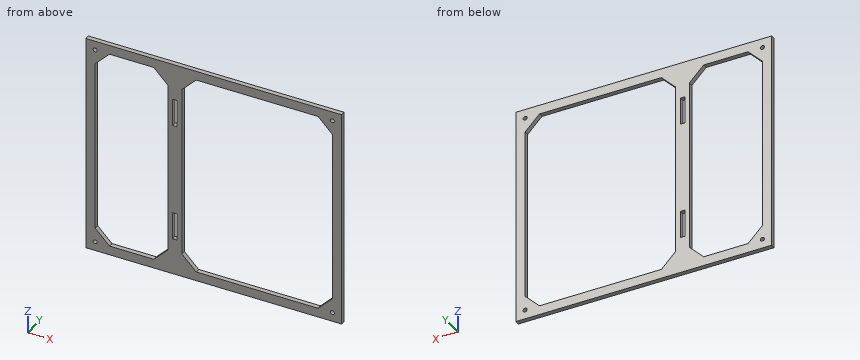
from build123d import *

# Parameters (mm, degrees)
SKETCH1_W           = 177.8
SKETCH1_H           = 152.4
SKETCH1_R           = 1.375
SKETCH1_W_2         = 3.175
SKETCH1_H_2         = 19.05
BOSS_EXTRUDE5_DEPTH = 3.175


with BuildPart() as part:
    # Sketch1 → Boss-Extrude5 (new body)
    with BuildSketch(Plane(origin=(0, 0, 0), x_dir=(1, 0, 0), z_dir=(0, 1, 0))):
        with Locations((88.9, 76.2)):
            Rectangle(SKETCH1_W, SKETCH1_H)
        with Locations(Location((6.35, 146.05, 0), (0, 0, 270))):
            Circle(SKETCH1_R, mode=Mode.SUBTRACT)
        with Locations(Location((6.35, 6.35, 0), (0, 0, 270))):
            Circle(SKETCH1_R, mode=Mode.SUBTRACT)
        with Locations(Location((171.45, 6.35, 0), (0, 0, 270))):
            Circle(SKETCH1_R, mode=Mode.SUBTRACT)
        with Locations(Location((171.45, 146.05, 0), (0, 0, 270))):
            Circle(SKETCH1_R, mode=Mode.SUBTRACT)
        Polygon((6.35, 16.35), (16.35, 6.35), (47.15, 6.35), (57.15, 16.35), (57.15, 136.05), (47.15, 146.05), (16.35, 146.05), (6.35, 136.05), align=None, mode=Mode.SUBTRACT)
        Polygon((76.675, 146.05), (161.45, 146.05), (171.45, 136.05), (171.45, 16.35), (161.45, 6.35), (76.675, 6.35), (66.675, 16.35), (66.675, 136.05), align=None, mode=Mode.SUBTRACT)
        with Locations((61.9125, 117.475)):
            Rectangle(SKETCH1_W_2, SKETCH1_H_2, mode=Mode.SUBTRACT)
        with Locations((61.9125, 34.925)):
            Rectangle(SKETCH1_W_2, SKETCH1_H_2, mode=Mode.SUBTRACT)
    extrude(amount=BOSS_EXTRUDE5_DEPTH)


solid = part.part
Model file for the job. Use its own axes, mm. Give positions to 0.01 mm unless a question says otherwise; leave off trailing zeros. Write each loop counter-clockwise with the first axis right and the second up, starting at its lowest first coordinate (ties: lowest second). Pieces come first, ordered by that corner, then holes. Notation, with made-up numbers: (3, 28.5) -> (57, 28.5) arc R16 cw to (57, 50.5) -> close; hole circle Ø6 at (0, 65). An arc over 180 degrees is marked (long way). Write item = value, one per line.
(1) Slice it at A-A, the plane z = -42. Give the cut face in (x, y) (3 decimals).
Determined:
outline = (0, 0) -> (6.35, 0) -> (6.35, 3.175) -> (0, 3.175) -> close; (57.15, 0) -> (60.325, 0) -> (60.325, 3.175) -> (57.15, 3.175) -> close; (63.5, 0) -> (66.675, 0) -> (66.675, 3.175) -> (63.5, 3.175) -> close; (171.45, 0) -> (177.8, 0) -> (177.8, 3.175) -> (171.45, 3.175) -> close
(2) Slice it at B-B, the plane y = 0.8. Give the number of separate pieces and of enclosed holes in the cut face, then the cut area to 3 significant figures.
Determined:
separate_pieces = 1
enclosed_holes = 8
area = 5,620 mm2
(3) Slice it at D-D, the plane z = -129.5. Give the cut face in (x, y) (3 decimals).
Determined:
outline = (0, 0) -> (6.35, 0) -> (6.35, 3.175) -> (0, 3.175) -> close; (57.15, 0) -> (66.675, 0) -> (66.675, 3.175) -> (57.15, 3.175) -> close; (171.45, 0) -> (177.8, 0) -> (177.8, 3.175) -> (171.45, 3.175) -> close
(4) Probe line 1 along Z through (x, y) = (61, 3.05); line 2 along X through (y, z) = (2.5, -123.5) (3 decimals); line 3 along X through (y, z) = (0.25, -76) (3 decimals). List the from-to ranges inside material, lowest first.
Determined:
line_1 = -152.4 to -127, -107.95 to -44.45, -25.4 to 0
line_2 = 0 to 6.35, 57.15 to 60.325, 63.5 to 66.675, 171.45 to 177.8
line_3 = 0 to 6.35, 57.15 to 66.675, 171.45 to 177.8
(5) Slice it at C-C, the plane x = 80.5. Give the cut face in (y, z) (3 decimals).
Determined:
outline = (0, -152.4) -> (3.175, -152.4) -> (3.175, -146.05) -> (0, -146.05) -> close; (0, -6.35) -> (3.175, -6.35) -> (3.175, 0) -> (0, 0) -> close
(6) Flat gauge pin, fed straight in: P1, Ø3, axis at x = 6.35, z = -146.05, coming from the +Y side (3 decimals). Where does the tip first touch, or does it go through?
Determined:
P1 = 3.175
